Check sheet for the modelled part. Datum: model origin and axes. Units: mm. A direction names the side the tool comes from. Round coordinates to 2 decimals unless told otherwise and drop trailing zeros. Write each loop counter-clockwise with the first axis right and the second up, starting at its lowest first coordinate (ties: lowest second). Pieces come first, ordered by that corner, then holes.
from build123d import *

# Parameters (mm, degrees)
AUFSATZ_LINEAR_AUSTRAGEN1_DEPTH = 26
SKIZZE2_R                       = 11
AUFSATZ_LINEAR_AUSTRAGEN2_DEPTH = 2
SKIZZE3_R                       = 2.5
AUFSATZ_LINEAR_AUSTRAGEN3_DEPTH = 26
SKIZZE4_R                       = 1.5
SCHNITT_LINEAR_AUSTRAGEN1_DEPTH = 4.5


with BuildPart() as part:
    # Skizze1 → Aufsatz-Linear austragen1 (new body)
    with BuildSketch(Plane(origin=(0, 0, 0), x_dir=(1, 0, 0), z_dir=(0, 1, 0))):
        Polygon((0, 37.8), (4.5, 42.3), (37.8, 42.3), (42.3, 37.8), (42.3, 4.5), (37.8, 0), (4.5, 0), (0, 4.5), align=None)
    extrude(amount=AUFSATZ_LINEAR_AUSTRAGEN1_DEPTH)

    # Skizze2 → Aufsatz-Linear austragen2 (add)
    with BuildSketch(Plane(origin=(0, 26, 0), x_dir=(1, 0, 0), z_dir=(0, 1, 0))):
        with Locations(Location((21.15, 21.15, 0), (0, 0, 270))):
            Circle(SKIZZE2_R)
    extrude(amount=AUFSATZ_LINEAR_AUSTRAGEN2_DEPTH)

    # Skizze3 → Aufsatz-Linear austragen3 (add)
    with BuildSketch(Plane(origin=(0, 28, 0), x_dir=(1, 0, 0), z_dir=(0, 1, 0))):
        with Locations(Location((21.15, 21.15, 0), (0, 0, 90))):
            Circle(SKIZZE3_R)
    extrude(amount=AUFSATZ_LINEAR_AUSTRAGEN3_DEPTH)

    # Skizze4 → Schnitt-Linear austragen1 (cut)
    with BuildSketch(Plane(origin=(0, 26, 0), x_dir=(1, 0, 0), z_dir=(0, 1, 0))):
        with Locations(Location((5.65, 36.65, 0), (0, 0, 270))):
            Circle(SKIZZE4_R)
        with Locations(Location((36.65, 36.65, 0), (0, 0, 270))):
            Circle(SKIZZE4_R)
        with Locations(Location((5.65, 5.65, 0), (0, 0, 90))):
            Circle(SKIZZE4_R)
        with Locations(Location((36.65, 5.65, 0), (0, 0, 90))):
            Circle(SKIZZE4_R)
    extrude(amount=-SCHNITT_LINEAR_AUSTRAGEN1_DEPTH, mode=Mode.SUBTRACT)


solid = part.part
1. Release check for a two-part mould opening along Z. For faces 1 (the flat face through (21, 54, -21)), 2 (the flat face through (6, 21.5, -6)), 3 (the cylindrical face through (22.11, 40.82, -23.46)), 4 (the flat face through (6, 21.5, -37)) record: released by +Z, released by -Z, zero draft, split by the parting line, or undercut.
2. Scan lines: line 1 along Z through (x, y) = (36, 22); line 2 along X through (y, z) = (23, -36); line 3 along Y through (x, z) = (26, -4). Record each from-to range of solid material in increasing order.
3. Sectioned sample at A-A, the plane z = -5.65. Enter the section's corners in (x, y).
4. Sectioned sample at C-C, the plane x = 36.65. Enter the section's corners in (y, z), plus the area to 3 significant figures.
5. Sectioned sample at B-B, the plane y = 24. Enter the section's corners in (x, z), plus the area to 3 significant figures.
6. Go/stop test with flat-tipped pins: pin 1 (2 mm diameter, centred on x = 25.5, z = -30.5, fed in from -Y); pin 2 (0.9 mm diameter, centred on x = 36, z = -36.5, fed in from +Y); pin 3 (12 mm diameter, centred on x = 19.5, z = -8, fed in from +Y); pin 4 (5 mm diameter, centred on x = 28.5, z = -9.5, fed in from +Y). Record where each tip stops, or that it passes through.
7. Set-up check for faces 5 (the flat face through (40.1, 12.8, -2.3)), 6 (the flat face through (37, 21.5, -37)): record each of +Z, -Z, +X, -X, +Y, -Y from which the full face is reachable in a straight line by a thin tool's end or side.
8. Sectioned sample at D-D, the plane y = 45. Enter the section's corners in (x, z), plus the area to 3 significant figures.
Computed values:
1. face 1: zero draft
1. face 2: undercut
1. face 3: split by the parting line
1. face 4: undercut
2. line 1: z = -42.3 to -38, -35.3 to -7, -4.3 to 0
2. line 2: x = 0 to 4.3, 7 to 35.3, 38 to 42.3
2. line 3: y = 0 to 26
3. outline: (0, 0) - (42.3, 0) - (42.3, 26) - (38.15, 26) - (38.15, 21.5) - (35.15, 21.5) - (35.15, 26) - (7.15, 26) - (7.15, 21.5) - (4.15, 21.5) - (4.15, 26) - (0, 26) - close
4. outline: (0, -42.3) - (26, -42.3) - (26, -38.15) - (21.5, -38.15) - (21.5, -35.15) - (26, -35.15) - (26, -7.15) - (21.5, -7.15) - (21.5, -4.15) - (26, -4.15) - (26, 0) - (0, 0) - close
4. area: 1,070 mm2
5. outline: (0, -37.8) - (4.5, -42.3) - (37.8, -42.3) - (42.3, -37.8) - (42.3, -4.5) - (37.8, 0) - (4.5, 0) - (0, -4.5) - close; hole circle Ø3 at (5.65, -36.65); hole circle Ø3 at (5.65, -5.65); hole circle Ø3 at (36.65, -36.65); hole circle Ø3 at (36.65, -5.65)
5. area: 1,720 mm2
6. pin 1: stops at y = 0
6. pin 2: stops at y = 21.5
6. pin 3: stops at y = 28
6. pin 4: stops at y = 26
7. face 5: +Z, +X, +Y, -Y
7. face 6: +Y
8. outline: circle Ø5 at (21.15, -21.15)
8. area: 19.6 mm2
